Geometry: final body of the model. Coordinates: model frame, mm. A direction names the side the tool comes from. Round coordinates to 2 decimals unless told otherwise and drop trailing zeros. Loops run counter-clockwise (first coordinate to the right, second up) from the corner with the lowest first, then second, coordinate; pieces in that order, holes last. Notation, with made-up numbers: M 51,89.25 L 103,89.25 A25 cw 103,128.25 Z; hole C 17.5,23 d6. An arc over 180 degrees is marked long. Return JSON: item names as keys, results as strings.
Autodesk Inventor part; units mm, degrees
ref_plane "Work Plane1" through (40, 10, 0) normal (0.7071, 0.7071, 0) x (0, 0, -1)
ref_plane "YZ Plane" through (0, 0, 0) normal (1, 0, 0) x (0, 1, 0)
ref_plane "XZ Plane" through (0, 0, 0) normal (0, 1, 0) x (-1, 0, 0)
sketch "Sketch1" plane through (0, 0, 0) normal (0, 1, 0) x (-1, 0, 0)
  line L0 (-40, 0) -> (-40, -100)
  line L1 (-30, -100) -> (-10, -100)
  line L2 (0, -10) -> (140, -10)
  line L3 (140, -90) -> (0, -90)
  arc A0 (0, 0) -> (-40, 0) centre (-20, 0) ccw
  arc A1 (-40, -100) -> (0, -100) centre (-20, -100) ccw
  circle A2 centre (-20, 0) radius 10
  circle A3 centre (-20, -100) radius 10
  arc A4 (120, -40) -> (120, -60) centre (120, -50) ccw
  line L4 (120, -40) -> (140, -40)
  line L5 (120, -60) -> (140, -60)
  line L6 (140, -10) -> (140, -40)
  line L7 (140, -60) -> (140, -90)
  line L8 (0, -100) -> (0, -90)
  line L9 (0, -10) -> (0, 0)
  line L10 (-30, 0) -> (-40, 0)
  dimension "d4" = 20
  dimension "d0" = 40
  dimension "d1" = 100
  dimension "d2" = 140
  dimension "d3" = 80
  dimension "d5" = 20
  dimension "d6" = 20
  dimension "d8" = 20
  dimension "d9" = 20
extrude "Extrusion1" add sketch "Sketch1" along normal blind 10
ref_plane "Work Plane1" through (40, 10, 0) normal (0.7071, 0.7071, 0) x (0, 0, -1)
sketch "Sketch2" plane through (0, 10, 0) normal (0, 1, 0) x (1, 0, 0)
  point P0 (0, 0)
sketch "Sketch3" plane through (40, 10, 0) normal (0.7071, 0.7071, 0) x (0, 0, -1)
  line L0 (90, 51) -> (90, 0)
  line L1 (90, 0) -> (10, 0)
  line L2 (10, 0) -> (10, 51)
  arc A0 (90, 51) -> (10, 51) centre (50, 51) ccw
  circle A1 centre (50, 51) radius 15
  point P0 (0, 21.2132)
  point P1 (90, 28.2843)
  dimension "d13" = 51
  dimension "d14" = 30
extrude "Extrusion2" add sketch "Sketch3" against normal up to next
sketch "Sketch4" plane through (40, 10, 0) normal (0.7071, 0.7071, 0) x (0, 0, -1)
  circle A0 centre (50, 51) radius 15
  circle A1 centre (50, 51) radius 15
  point P0 (0, 21.2132)
  dimension "d17" = 30
extrude "Extrusion3" cut sketch "Sketch4" against normal up to surface surface through (-48.5464, 0, -50) normal (0, 1, 0)
properties part number "BT2" material "Nylon 6/6"
Q1. Pull-direction query (Y, two-part tool) for faces 6 (the flat face through (-30, 11, -10)), 7 (the flat face through (15, 35, -58)), 8 (the cylindrical face through (-28.234, 34.924, -48.047)); classes: pulls with the +Y half, pulls with the -Y half, needs draft (parallel to the pull), parting line crosses it, or undercut.
Determined:
{"face 6": "needs draft", "face 7": "pulls with the +Y half", "face 8": "undercut"}
Q2. Reachability of faces 1 (the flat face through (20, 10, 12)), 2 (the flat face through (20, 10, -111)), 3 (the flat face through (-130, 5, -40)), 4 (the flat face through (0, 5, -5)), 5 (the cylindrical face through (-48.95, 49.73, -50.88)) from +Z, -Z, +X, -X, +Y, -Y: full face, straight path, thin tool, end or side. Return the list, or none.
Determined:
{"face 1": "+Z, +X, -X, +Y", "face 2": "-Z, +X, -X, +Y", "face 3": "-X, +Y, -Y", "face 4": "+Z, -X, +Y, -Y", "face 5": "-X, +Y"}
Q3. Pin query (flat end, axial travel): pin 1 (14 mm diameter, centred on x = -76, y = 18, fed in from +Z); pin 2 (8 mm diameter, centred on x = -129.5, y = 6.5, fed in from -Z); pin 3 (6 mm diameter, centred on x = -49.5, z = -6.5, fed in from -Y); pin 4 (3 mm diameter, centred on y = 6.5, z = -93, fed in from -X). Return the tip coordinate at first contact, or that it passes through.
Determined:
{"pin 1": "stops at z = -23.19", "pin 2": "stops at z = -90", "pin 3": "passes through", "pin 4": "stops at x = 0"}
Q4. Section query C-C (y = 6). State how many separate pieces and enclosed holes the cut face has, plus the area to 3 significant figures.
Determined:
{"separate pieces": "1", "enclosed holes": "3", "area": "14,300 mm^2"}
Q5. Section query B-B (z = -81.5). Output: boundary loops of the cut face in (x, y), plus the area to 3 significant figures.
Determined:
{"outline": "M -140,0 L 40,0 L 40,10 L -13.49,63.49 L -66.99,10 L -140,10 Z", "area": "4,660 mm^2"}
Q6. Section query A-A (z = -50). Output: boundary loops of the cut face in (x, y).
Determined:
{"outline": "M -110,0 L -63.34,0 L -6.67,56.67 L -24.35,74.35 L -88.69,10 L -110,10 Z; M -20.91,0 L 40,0 L 40,10 L 14.54,35.46 Z"}
Q7. Material intervals for L1, parallel to Z at x = 20, y = 2; L2, parallel to X at y = 7, z = 0; L3, parallel to Y at x = -65, z = -14, sorted ascending.
Determined:
{"L1": "z = -120 to -110, -90 to -10, 10 to 20", "L2": "x = 0 to 10, 30 to 40", "L3": "y = 0 to 10"}
